```python
from build123d import *

# Parameters (mm, degrees)
F3_DEPTH      = 182.88
F3_DEPTH_BACK = 182.88
F4_W          = 43.18
F4_H          = 292.1
F4_H_2        = 12.7
F6_DEPTH      = 365.761
F9_DEPTH      = 304.801
F7_W          = 208.28
F7_H          = 81.28
F10_DEPTH     = 279.4
F11_SIZE      = 12.7
F12_SCALE     = 0.0393700787
F13_DEPTH     = 1
F14_SIZE      = 2


with BuildPart() as f1:
    # F0 (on Top) → F1 (revolve)
    with BuildSketch(Plane.XY):
        Polygon((182.88, 231.14), (-182.88, 231.14), (-182.88, 101.6), (421.64, 101.6), (421.64, 304.8), (182.88, 304.8), align=None)
    revolve(axis=Axis((286.554813385, 0, 0), (1, 0, 0)))

    # F2 (on Right) → F3 (cut, two sides)
    with BuildSketch(Plane.YZ) as f3_sk:
        with BuildLine():
            Line((-46.7577635634, 189.9085252076), (-48.6472827621, 225.9626993109))
            ThreePointArc((-48.6472827621, 225.9626993109), (-71.4261880798, 219.8272031765), (-93.4610637385, 211.401819209))
            Line((-93.4610637385, 211.401819209), (-73.7976050599, 181.1227481224))
            ThreePointArc((-73.7976050599, 181.1227481224), (-60.4375437599, 186.007633457), (-46.7577635634, 189.9085252076))
        make_face()
        with BuildLine():
            Line((14.2156859414, 195.0626839588), (23.559998911, 229.9361347229))
            ThreePointArc((23.559998911, 229.9361347229), (0, 231.14), (-23.559998911, 229.9361347229))
            Line((-23.559998911, 229.9361347229), (-14.2156859414, 195.0626839588))
            ThreePointArc((-14.2156859414, 195.0626839588), (0, 195.58), (14.2156859414, 195.0626839588))
        make_face()
        with BuildLine():
            ThreePointArc((93.4610637385, 211.401819209), (71.4261880798, 219.8272031765), (48.6472827621, 225.9626993109))
            Line((48.6472827621, 225.9626993109), (46.7577635634, 189.9085252076))
            ThreePointArc((46.7577635634, 189.9085252076), (60.4375437599, 186.007633457), (73.7976050599, 181.1227481224))
            Line((73.7976050599, 181.1227481224), (93.4610637385, 211.401819209))
        make_face()
        with BuildLine():
            ThreePointArc((154.2135084657, 172.1740207078), (135.8606832149, 186.9961880798), (116.0926294528, 199.8704605156))
            Line((116.0926294528, 199.8704605156), (103.1542373903, 166.1647968387))
            ThreePointArc((103.1542373903, 166.1647968387), (114.9590396434, 158.2275437599), (126.1557004169, 149.4532557435))
            Line((126.1557004169, 149.4532557435), (154.2135084657, 172.1740207078))
        make_face()
        with BuildLine():
            ThreePointArc((199.8704605156, 116.0926294528), (186.9961880798, 135.8606832149), (172.1740207078, 154.2135084657))
            Line((172.1740207078, 154.2135084657), (149.4532557435, 126.1557004169))
            ThreePointArc((149.4532557435, 126.1557004169), (158.2275437599, 114.9590396434), (166.1647968387, 103.1542373903))
            Line((166.1647968387, 103.1542373903), (199.8704605156, 116.0926294528))
        make_face()
        with BuildLine():
            ThreePointArc((225.9626993109, 48.6472827621), (219.8272031765, 71.4261880798), (211.401819209, 93.4610637385))
            Line((211.401819209, 93.4610637385), (181.1227481224, 73.7976050599))
            ThreePointArc((181.1227481224, 73.7976050599), (186.007633457, 60.4375437599), (189.9085252076, 46.7577635634))
            Line((189.9085252076, 46.7577635634), (225.9626993109, 48.6472827621))
        make_face()
        with BuildLine():
            ThreePointArc((231.14, 0), (230.8388374818, 11.7953681618), (229.9361347229, 23.559998911))
            Line((229.9361347229, 23.559998911), (195.0626839588, 14.2156859414))
            ThreePointArc((195.0626839588, 14.2156859414), (195.4506282014, 7.1125477621), (195.58, 0))
            ThreePointArc((195.58, 0), (195.4506282014, -7.1125477621), (195.0626839588, -14.2156859414))
            Line((195.0626839588, -14.2156859414), (229.9361347229, -23.559998911))
            ThreePointArc((229.9361347229, -23.559998911), (230.8388374818, -11.7953681618), (231.14, 0))
        make_face()
        with BuildLine():
            ThreePointArc((211.401819209, -93.4610637385), (219.8272031765, -71.4261880798), (225.9626993109, -48.6472827621))
            Line((225.9626993109, -48.6472827621), (189.9085252076, -46.7577635635))
            ThreePointArc((189.9085252076, -46.7577635635), (186.007633457, -60.4375437599), (181.1227481224, -73.7976050599))
            Line((181.1227481224, -73.7976050599), (211.401819209, -93.4610637385))
        make_face()
        with BuildLine():
            ThreePointArc((172.1740207078, -154.2135084657), (186.9961880798, -135.8606832149), (199.8704605156, -116.0926294528))
            Line((199.8704605156, -116.0926294528), (166.1647968387, -103.1542373903))
            ThreePointArc((166.1647968387, -103.1542373903), (158.2275437599, -114.9590396434), (149.4532557435, -126.1557004169))
            Line((149.4532557435, -126.1557004169), (172.1740207078, -154.2135084657))
        make_face()
        with BuildLine():
            ThreePointArc((116.0926294528, -199.8704605156), (135.8606832149, -186.9961880798), (154.2135084657, -172.1740207078))
            Line((154.2135084657, -172.1740207078), (126.1557004169, -149.4532557435))
            ThreePointArc((126.1557004169, -149.4532557435), (114.9590396434, -158.2275437599), (103.1542373903, -166.1647968387))
            Line((103.1542373903, -166.1647968387), (116.0926294528, -199.8704605156))
        make_face()
        with BuildLine():
            ThreePointArc((48.6472827621, -225.9626993109), (71.4261880798, -219.8272031765), (93.4610637385, -211.401819209))
            Line((93.4610637385, -211.401819209), (73.7976050599, -181.1227481224))
            ThreePointArc((73.7976050599, -181.1227481224), (60.4375437599, -186.007633457), (46.7577635634, -189.9085252076))
            Line((46.7577635634, -189.9085252076), (48.6472827621, -225.9626993109))
        make_face()
        with BuildLine():
            ThreePointArc((-23.559998911, -229.9361347229), (0, -231.14), (23.559998911, -229.9361347229))
            Line((23.559998911, -229.9361347229), (14.2156859414, -195.0626839588))
            ThreePointArc((14.2156859414, -195.0626839588), (0, -195.58), (-14.2156859414, -195.0626839588))
            Line((-14.2156859414, -195.0626839588), (-23.559998911, -229.9361347229))
        make_face()
        with BuildLine():
            Line((-73.7976050599, -181.1227481224), (-93.4610637385, -211.401819209))
            ThreePointArc((-93.4610637385, -211.401819209), (-71.4261880798, -219.8272031765), (-48.6472827621, -225.9626993109))
            Line((-48.6472827621, -225.9626993109), (-46.7577635635, -189.9085252076))
            ThreePointArc((-46.7577635635, -189.9085252076), (-60.4375437599, -186.007633457), (-73.7976050599, -181.1227481224))
        make_face()
        with BuildLine():
            Line((-126.1557004169, -149.4532557435), (-154.2135084657, -172.1740207078))
            ThreePointArc((-154.2135084657, -172.1740207078), (-135.8606832149, -186.9961880798), (-116.0926294528, -199.8704605156))
            Line((-116.0926294528, -199.8704605156), (-103.1542373903, -166.1647968387))
            ThreePointArc((-103.1542373903, -166.1647968387), (-114.9590396434, -158.2275437599), (-126.1557004169, -149.4532557435))
        make_face()
        with BuildLine():
            Line((-166.1647968387, -103.1542373903), (-199.8704605156, -116.0926294528))
            ThreePointArc((-199.8704605156, -116.0926294528), (-186.9961880798, -135.8606832149), (-172.1740207078, -154.2135084657))
            Line((-172.1740207078, -154.2135084657), (-149.4532557435, -126.1557004169))
            ThreePointArc((-149.4532557435, -126.1557004169), (-158.2275437599, -114.9590396434), (-166.1647968387, -103.1542373903))
        make_face()
        with BuildLine():
            Line((-189.9085252076, -46.7577635634), (-225.9626993109, -48.6472827621))
            ThreePointArc((-225.9626993109, -48.6472827621), (-219.8272031765, -71.4261880798), (-211.401819209, -93.4610637385))
            Line((-211.401819209, -93.4610637385), (-181.1227481224, -73.7976050599))
            ThreePointArc((-181.1227481224, -73.7976050599), (-186.007633457, -60.4375437599), (-189.9085252076, -46.7577635634))
        make_face()
        with BuildLine():
            Line((-195.0626839588, 14.2156859414), (-229.9361347229, 23.559998911))
            ThreePointArc((-229.9361347229, 23.559998911), (-231.14, 0), (-229.9361347229, -23.559998911))
            Line((-229.9361347229, -23.559998911), (-195.0626839588, -14.2156859414))
            ThreePointArc((-195.0626839588, -14.2156859414), (-195.58, 0), (-195.0626839588, 14.2156859414))
        make_face()
        with BuildLine():
            Line((-181.1227481224, 73.7976050599), (-211.401819209, 93.4610637385))
            ThreePointArc((-211.401819209, 93.4610637385), (-219.8272031765, 71.4261880798), (-225.9626993109, 48.6472827621))
            Line((-225.9626993109, 48.6472827621), (-189.9085252076, 46.7577635634))
            ThreePointArc((-189.9085252076, 46.7577635635), (-186.007633457, 60.4375437599), (-181.1227481224, 73.7976050599))
        make_face()
        with BuildLine():
            Line((-149.4532557435, 126.1557004169), (-172.1740207078, 154.2135084657))
            ThreePointArc((-172.1740207078, 154.2135084657), (-186.9961880798, 135.8606832149), (-199.8704605156, 116.0926294528))
            Line((-199.8704605156, 116.0926294528), (-166.1647968387, 103.1542373903))
            ThreePointArc((-166.1647968387, 103.1542373903), (-158.2275437599, 114.9590396434), (-149.4532557435, 126.1557004169))
        make_face()
        with BuildLine():
            Line((-103.1542373903, 166.1647968387), (-116.0926294528, 199.8704605156))
            ThreePointArc((-116.0926294528, 199.8704605156), (-135.8606832149, 186.9961880798), (-154.2135084657, 172.1740207078))
            Line((-154.2135084657, 172.1740207078), (-126.1557004169, 149.4532557435))
            ThreePointArc((-126.1557004169, 149.4532557435), (-114.9590396434, 158.2275437599), (-103.1542373903, 166.1647968387))
        make_face()
    extrude(amount=-F3_DEPTH, mode=Mode.SUBTRACT)
    extrude(f3_sk.sketch, amount=F3_DEPTH_BACK, mode=Mode.SUBTRACT)

    # F4 (on Top) → F5 (revolve)
    with BuildSketch(Plane.XY):
        Polygon((-139.7, 0), (-182.88, 0), (-182.88, -14.2156859414), (-182.88, -292.1), (-139.7, -292.1), align=None)
        with Locations((161.29, -146.05)):
            Rectangle(F4_W, F4_H)
        with Locations((161.29, -298.45)):
            Rectangle(F4_W, F4_H_2)
    revolve(axis=Axis((-161.29, 0, 0), (-1, 0, 0)))

    # F6 (cut, through all): a face of the model
    f6_faces = [f1.faces().sort_by_distance(p)[0] for p in [
        (182.88, 0, 0),
    ]]
    extrude(f6_faces, amount=-F6_DEPTH, mode=Mode.SUBTRACT)

    # F8 (on Top) → F9 (cut, through all)
    with BuildSketch(Plane.XY):
        with BuildLine():
            Line((217.17, 0), (318.77, 0))
            ThreePointArc((318.77, 0), (267.97, 50.8), (217.17, 0))
        make_face()
        with BuildLine():
            ThreePointArc((217.17, 0), (267.97, -50.8), (318.77, 0))
            Line((318.77, 0), (217.17, 0))
        make_face()
    extrude(amount=F9_DEPTH, mode=Mode.SUBTRACT)

    # F7 (on face) → F10 (cut)
    with BuildSketch(Plane.YZ.offset(421.64)):
        with Locations((0, 171.45)):
            Rectangle(F7_W, F7_H)
    extrude(amount=-F10_DEPTH, mode=Mode.SUBTRACT)

    # F11
    f11_edges = [f1.edges().sort_by_distance(p)[0] for p in [
        (281.94, -104.14, 212.09),
        (281.94, 104.14, 212.09),
    ]]
    chamfer(f11_edges, length=F11_SIZE)


with BuildPart() as f1_1:
    # F12: moved
    add(f1.part.scale(F12_SCALE))

    # F13 (add): a face of the model
    f13_faces = [f1_1.faces().sort_by_distance(p)[0] for p in [
        (-7.2, 11.1747308807, 0),
    ]]
    extrude(f13_faces, amount=F13_DEPTH)

    # F14
    f14_edges = [f1_1.edges().sort_by_distance(p)[0] for p in [
        (-5.5, 11.5, 0),
    ]]
    chamfer(f14_edges, length=F14_SIZE)


solid = f1_1.part
```
Geometry: final body of the model. Coordinates: model frame, mm. A direction names the side the tool comes from. Give positions to 0.01 mm unless a question says otherwise; leave off trailing zeros. Order: outer loops, then holes, each group sorted by start corner. A loop starts at its lowest first (then second) coordinate and runs counter-clockwise, first axis right, second up. Notation, with made-up numbers: (-18.5, 13) -> (28.5, 13) arc R21 ccw to (28.5, 23) -> close; hole circle Ø6 at (33.5, 51). An arc over 180 degrees is marked (long way). Write each question's results on one line, items separated by ' | '. Start each with the question number.
1) Set-up query: faces 1 (the cylindrical face through (-0.08, -8.11, -4.13)), 2 (the cylindrical face through (12.548, -0.088, 4.483)), 3 (the cylindrical face through (-0.077, 8.987, -1.43)), 4 (the flat face through (-0.08, 7.74, 3.3)). Return all of +Z, -Z, +X, -X, +Y, -Y with unobstructed straight access to the full face (end or side cutting, diameter ignored); none if empty.
2) Section C-C (x = 10.55). Return loops of the section in (y, z), then the cut area to 3 significant figures.
3) Line query: line 1 (X direction, y = 8.5, z = 3); line 2 (Y direction, x = 0.75, z = 7.5); line 3 (X direction, y = 0, z = 10). Output: solid intervals per line, ascending. Write a range as from..to.
4) Section A-A (z = 0). Return loops of the section in (x, y), then the cut area to 4 significant figures.
5) First-contact query: pin 1 (2 mm diameter, centred on x = 6.5, y = -1.5, fed in from +Z); pin 2 (5 mm diameter, centred on x = -1, y = -4, fed in from -Z); pin 3 (5 mm diameter, centred on x = 9.5, y = -4.5, fed in from -Z); pin 4 (6.5 mm diameter, centred on y = 0, z = 0, fed in from -X). Flat tips, straight axial feed; report the tip coordinate or a pass-through.
6) Draft query along Y for faces 5 (the flat face through (0.077, -6.325, 5.511)), 6 (the flat face through (-0.077, 7.215, -4.319)), 7 (the conical face through (-6, 8, -6)), 8 (the cylindrical face through (-0.077, -6.225, -4.532)). Return one class per face: pulls with the +Y half, pulls with the -Y half, needs draft (parallel to the pull), parting line crosses it, or undercut.
7) Section B-B (y = 0). Count the separate pieces of the cut face and the enclosed holes in it, then the cut area to 3 significant figures.
Calculated:
1) face 1: -Z, -Y | face 2: +Z | face 3: -Z, +Y | face 4: +Y
2) outline: (-4.1, 5.15) -> (-4.1, 7.85) -> (-3.6, 8.35) -> (-2, 8.35) -> (-2, 11.83) arc R12 ccw (long way) to (2, 11.83) -> (2, 8.35) -> (3.6, 8.35) -> (4.1, 7.85) -> (4.1, 5.15) -> (2, 5.15) -> (2, 3.46) arc R4 cw (long way) to (-2, 3.46) -> (-2, 5.15) -> close | area: 356 mm2
3) line 1: -8.2..-5.5, 5.5..16.6 | line 2: -4.43..-3.15, -1.84..1.84, 3.15..4.43 | line 3: -8.2..-6, 5.5..8.55, 12.55..16.6
4) outline: (-8.2, -11.5) -> (-7.5, -11.5) -> (-5.5, -9.5) -> (-5.5, -7.7) -> (5.5, -7.7) -> (5.5, -12) -> (16.6, -12) -> (16.6, -4) -> (-8.2, -4) -> close; (-8.2, 4) -> (16.6, 4) -> (16.6, 12) -> (5.5, 12) -> (5.5, 7.7) -> (-5.5, 7.7) -> (-5.5, 9.5) -> (-7.5, 11.5) -> (-8.2, 11.5) -> close | area: 295.5 mm2
5) pin 1: z = 11.99 | pin 2: z = -8.98 | pin 3: z = -11.83 | pin 4: through
6) face 5: pulls with the -Y half | face 6: undercut | face 7: parting line crosses it | face 8: undercut
7) separate pieces: 4 | enclosed holes: 0 | area: 241 mm2
